from build123d import *

# Parameters (mm, degrees)
SKETCH_1_R               = 2.5
EXTRUDE_1_DEPTH          = 1.5
SKETCH_3_R               = 3.05
EXTRUDE_2_DEPTH          = 0.5
SKETCH_4_R               = 1
CUT_EXTRUDE_1_DEPTH      = 1
CUT_EXTRUDE_1_DEPTH_BACK = 2.5


with BuildPart() as part:
    # Эскиз1 → Бобышка-Вытянуть1 (new body)
    with BuildSketch(Plane.XY):
        Circle(SKETCH_1_R)
    extrude(amount=EXTRUDE_1_DEPTH)

    # Эскиз3 → Бобышка-Вытянуть2 (add)
    with BuildSketch(Plane(origin=(0, 0, 0), x_dir=(-1, 0, 0), z_dir=(0, 0, -1))):
        Circle(SKETCH_3_R)
    extrude(amount=-EXTRUDE_2_DEPTH)

    # Эскиз4 → Вырез-Вытянуть1 (cut, two sides)
    with BuildSketch(Plane.XY.offset(1.5)) as cut_extrude_1_sk:
        Circle(SKETCH_4_R)
    extrude(amount=CUT_EXTRUDE_1_DEPTH, mode=Mode.SUBTRACT)
    extrude(cut_extrude_1_sk.sketch, amount=-CUT_EXTRUDE_1_DEPTH_BACK, mode=Mode.SUBTRACT)


solid = part.part
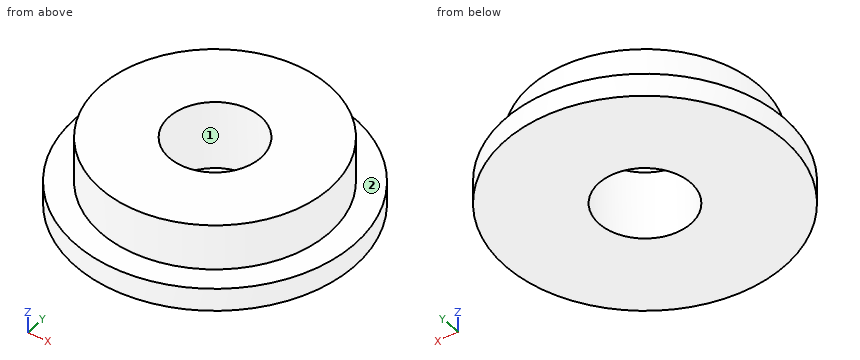
Could you check a few things on this model? Use its own coordinates, in mm. Face numbers are marked on the shaded views. A direction names the side the tool comes from. Round coordinates to 2 decimals unless told otherwise and drop trailing zeros. Loops run counter-clockwise (first coordinate to the right, second up) from the corner with the lowest first, then second, coordinate; pieces in that order, holes last. Notation, with made-up numbers: (30.25, 89.5) -> (56.25, 89.5) arc R7 ccw to (56.25, 100.5) -> close; hole circle Ø5 at (57.5, -39). An arc over 180 degrees is marked (long way). Use CSV: the item, a comma, the result in double quotes.
(1) Suppose I cut it at D-D on y = -2. Write out the boundary of the cut face in (x, z).
Return value:
outline,"(-2.3, 0) -> (2.3, 0) -> (2.3, 0.5) -> (1.5, 0.5) -> (1.5, 1.5) -> (-1.5, 1.5) -> (-1.5, 0.5) -> (-2.3, 0.5) -> close"
(2) For the marked faces 1 and 2, which set-ups out of +Z, -Z, +X, -X, +Y, -Y let a thin tool reach every point of the face, with its end or its side?
Return value:
face 1,"+Z, -Z"
face 2,"+Z"
(3) Will this pin go through, and if not, where does the flat tip stop? pin 1 Ø1.5 at (x, y) = (1, 0) entering from -Z.
Return value:
pin 1,"stops at z = 0"
(4) If I drill on probe 1 along Y at (x, z) = (0, 1.05); probe 2 along Y at (x, z) = (0, 0.45); probe 3 along Z at (x, y) = (-2, -2), over which ranges is the centre line in solid material (lowest first)? Write a range as [from, to].
Return value:
probe 1,"y = [-2.5, -1], [1, 2.5]"
probe 2,"y = [-3.05, -1], [1, 3.05]"
probe 3,"z = [0, 0.5]"
(5) Suppose I cut it at A-A on y = 0. Write out the boundary of the cut face in (x, z), plus the area to 3 significant figures.
Return value:
outline,"(-3.05, 0) -> (-1, 0) -> (-1, 1.5) -> (-2.5, 1.5) -> (-2.5, 0.5) -> (-3.05, 0.5) -> close; (1, 0) -> (3.05, 0) -> (3.05, 0.5) -> (2.5, 0.5) -> (2.5, 1.5) -> (1, 1.5) -> close"
area,"5.05 mm²"
(6) Suppose I cut it at C-C on z = 0.75. Write out the boundary of the cut face in (x, y).
Return value:
outline,"circle Ø5 at (0, 0); hole circle Ø2 at (0, 0)"
